from build123d import *

# Parameters (mm, degrees)
SKETCH1_R               = 68
BOSS_EXTRUDE1_DEPTH     = 115
SHELL1_T                = 5
FILLET1_R               = 5
CUT_EXTRUDE1_DEPTH      = 159.297188857
CUT_EXTRUDE1_DEPTH_BACK = 159.297188857
SKETCH2_R               = 40
FILLET3_R               = 2.5


# Some blends are built 0.0001 mm under size
with BuildPart() as part:
    # Sketch1 → Boss-Extrude1 (new body)
    with BuildSketch(Plane(origin=(0, 0, 0), x_dir=(1, 0, 0), z_dir=(0, 1, 0))):
        with Locations(Location((0, 0, 0), (0, 0, 270))):
            Circle(SKETCH1_R)
    extrude(amount=BOSS_EXTRUDE1_DEPTH)

    # Shell1
    shell1_openings = [part.faces().sort_by_distance(p)[0] for p in [
        (0, 115, 0),
    ]]
    offset(amount=SHELL1_T, openings=shell1_openings, kind=Kind.INTERSECTION)

    # Fillet1
    # the kernel refuses this fillet: 5 mm, written as the material it takes off along each edge
    with BuildSketch(Plane(origin=(0, -5, 0), x_dir=(0, 0, 1), z_dir=(1, 0, 0))) as fillet1_piece_1:
        with BuildLine():
            CenterArc((73 - FILLET1_R, -FILLET1_R), FILLET1_R, 0, 90)
            Line((73 - FILLET1_R, 0), (73, 0))
            Line((73, 0), (73, -FILLET1_R))
        make_face()
    revolve(axis=Axis((0, -5, 0), (0, -1, 0)), mode=Mode.SUBTRACT)

    # Sketch2 → Cut-Extrude1 (cut, two sides: drawn at the far end of the back side and taken through both)
    with BuildSketch(Plane.XZ.offset(5).offset(-CUT_EXTRUDE1_DEPTH_BACK)):
        with Locations(Location((0, 0, 0), (0, 0, 270))):
            Circle(SKETCH2_R)
    extrude(amount=CUT_EXTRUDE1_DEPTH + CUT_EXTRUDE1_DEPTH_BACK, mode=Mode.SUBTRACT)

    # Fillet3
    fillet3_edges = [part.edges().sort_by_distance(p)[0] for p in [
        (0, -5, 40),
        (0, 0, 40),
    ]]
    fillet(fillet3_edges, radius=FILLET3_R - 0.0001)  # a hair under: the kernel refuses the full size


solid = part.part
Source: CAD feature listing. Evaluate the final solid. Frame: model axes, mm. A direction names the side the tool comes from. Coordinates: 2 decimals unless noted, no trailing zeros. Loops run counter-clockwise (first coordinate to the right, second up) from the corner with the lowest first, then second, coordinate; pieces in that order, holes last. Notation, with made-up numbers: M 88.5,57.5 L 118.5,57.5 A23 ccw 118.5,81.5 Z; hole C -12.75,70 d7. An arc over 180 degrees is marked long. Answer in a Markdown table with one row per item.
Q1. First-contact query: pin 1 (6 mm diameter, centred on x = 54.5, z = 4, fed in from +Y); pin 2 (12 mm diameter, centred on x = 23.5, y = 13, fed in from -Z); pin 3 (8 mm diameter, centred on y = 50.5, z = -50, fed in from +X). Flat tips, straight axial feed; report the tip coordinate or a pass-through.
Answers below:
| item | result |
|---|---|
| pin 1 | stops at y = 0 |
| pin 2 | stops at z = -70.87 |
| pin 3 | stops at x = 56.68 |
Q2. Set-up query: faces 4 (the flat face through (31.2, -5, 29.3)), 5 (the flat face through (31.2, 0, 29.3)). Return all of +Z, -Z, +X, -X, +Y, -Y with unobstructed straight access to the full face (end or side cutting, diameter ignored); none if empty.
Answers below:
| item | result |
|---|---|
| face 4 | +Z, -Z, +X, -X, -Y |
| face 5 | +Y |
Q3. Ray query, probe 1 along X at (y, z) = (90, 0); probe 2 along Y at (x, z) = (10, 51). Return the intervals inside material, ascending. Write a range as from..to.
Answers below:
| item | result |
|---|---|
| probe 1 | x = -73..-68, 68..73 |
| probe 2 | y = -5..0 |
Q4. Section C-C on y = 21.5. Return the cut outline in (x, z).
Answers below:
| item | result |
|---|---|
| outline | C 0,0 d146; hole C 0,0 d136 |
Q5. Draft query along Z for faces 1 (the cylindrical face through (67.42, 56.7, -8.85)), 2 (the cylindrical face through (-71.264, 56.695, -15.825)), 3 (the flat face through (33, 115, -60)). Return one class per face: pulls with the +Z half, pulls with the -Z half, needs draft (parallel to the pull), parting line crosses it, or undercut.
Answers below:
| item | result |
|---|---|
| face 1 | undercut |
| face 2 | parting line crosses it |
| face 3 | needs draft |
